from build123d import *

# Parameters (mm, degrees)
SKETCH1_R                                            = 166
SKETCH1_R_2                                          = 131
BOSS_EXTRUDE1_DEPTH                                  = 15
M6_CLEARANCE_HOLE1_D                                 = 6.6
CIRPATTERN1_COUNT                                    = 8
SKETCH4_R                                            = 10
CUT_EXTRUDE1_DEPTH                                   = 4
CSK_FOR_M10_HEX_SOCKET_COUNTERSUNK_CAP_S_D           = 11
CSK_FOR_M10_HEX_SOCKET_COUNTERSUNK_CAP_S_CSINK_D     = 24.4
CSK_FOR_M10_HEX_SOCKET_COUNTERSUNK_CAP_S_CSINK_ANGLE = 90
CIRPATTERN2_COUNT                                    = 4


with BuildPart() as part:
    # Sketch1 → Boss-Extrude1 (new body)
    with BuildSketch(Plane(origin=(0, 0, 0), x_dir=(1, 0, 0), z_dir=(0, 1, 0))):
        Circle(SKETCH1_R)
        Circle(SKETCH1_R_2, mode=Mode.SUBTRACT)
    extrude(amount=BOSS_EXTRUDE1_DEPTH)

    # M6 Clearance Hole1 (through all)
    with Locations(Plane(origin=(0, 0, 0), x_dir=(-1, 0, 0), z_dir=(0, -1, 0))):
        with Locations((0, 153)):
            m6_clearance_hole1 = Hole(M6_CLEARANCE_HOLE1_D / 2)

    # CirPattern1: M6 Clearance Hole1 ×8 about axis
    cirpattern1_axis = Axis((0, 0, 0), (0, 1, 0))
    for i in range(1, CIRPATTERN1_COUNT):
        add(m6_clearance_hole1.rotate(cirpattern1_axis, i * 360 / CIRPATTERN1_COUNT), mode=Mode.SUBTRACT)

    # Sketch4 → Cut-Extrude1 (cut)
    with BuildSketch(Plane.XZ):
        with Locations((-137.196110578, 56.828489706)):
            Circle(SKETCH4_R)
    cut_extrude1 = extrude(amount=-CUT_EXTRUDE1_DEPTH, mode=Mode.SUBTRACT)

    # CSK for M10 Hex Socket Countersunk Cap Screw1 (through all)
    with Locations(Plane(origin=(0, 15, 0), x_dir=(1, 0, 0), z_dir=(0, 1, 0))):
        with Locations((-137.196110578, -56.828489706)):
            csk_for_m10_hex_socket_countersunk_cap_s = CounterSinkHole(CSK_FOR_M10_HEX_SOCKET_COUNTERSUNK_CAP_S_D / 2, CSK_FOR_M10_HEX_SOCKET_COUNTERSUNK_CAP_S_CSINK_D / 2, counter_sink_angle=CSK_FOR_M10_HEX_SOCKET_COUNTERSUNK_CAP_S_CSINK_ANGLE)

    # CirPattern2: Cut-Extrude1, CSK for M10 Hex Socket Countersunk Cap Screw1 ×4 about axis
    cirpattern2_axis = Axis((0, 0, 0), (0, 1, 0))
    for i in range(1, CIRPATTERN2_COUNT):
        add(cut_extrude1.rotate(cirpattern2_axis, i * 360 / CIRPATTERN2_COUNT), mode=Mode.SUBTRACT)
        add(csk_for_m10_hex_socket_countersunk_cap_s.rotate(cirpattern2_axis, i * 360 / CIRPATTERN2_COUNT), mode=Mode.SUBTRACT)


solid = part.part
Geometry check sheet. Reference: the model listing, model coordinates, mm. A direction names the side the tool comes from. Give positions to 0.01 mm unless a question says otherwise; leave off trailing zeros. Order: outer loops, then holes, each group sorted by start corner. A loop starts at its lowest first (then second) coordinate and runs counter-clockwise, first axis right, second up. Notation, with made-up numbers: M -26.5,13 L 29.5,13 A18 cw 29.5,26 Z; hole C 88,78 d9. An arc over 180 degrees is marked long. Use a Markdown table: item, result.
Item 1: Material ranges on line 1 along X through (y, z) = (9.5, 0); line 2 along Z through (x, y) = (107, 13.25); line 3 along Z through (x, y) = (-153, 10), recorded low to high.
Answers follow:
| item | result |
|---|---|
| line 1 | x = -166 to -156.3, -149.7 to -131, 131 to 149.7, 156.3 to 166 |
| line 2 | z = -126.91 to -111.27, -105.11 to -75.58, 75.58 to 105.11, 111.27 to 126.91 |
| line 3 | z = -64.4 to -3.3, 3.3 to 64.4 |
Item 2: Section check B-B (z = 77). Record the cut outline in (x, y).
Answers follow:
| item | result |
|---|---|
| outline | M -147.06,0 L -105.98,0 L -105.98,15 L -147.06,15 Z; M 105.98,0 L 147.06,0 L 147.06,15 L 105.98,15 Z |
Item 3: Depth check by flat-ended pin: P1, Ø14.5, axis at x = 137.2, z = -56.83, coming from the +Y side; P2, Ø10.5, axis at x = 108.19, z = 108.19, coming from the -Y side; P3, Ø5, axis at y = 1.5, z = 40, coming from the -X side; P4, Ø3, axis at x = -126.5, y = 13, coming from the -Z side. Enter the tip coordinate at first touch or a pass-through.
Answers follow:
| item | result |
|---|---|
| P1 | stops at y = 10.05 |
| P2 | stops at y = 0 |
| P3 | stops at x = -161.71 |
| P4 | stops at z = -109.23 |
Item 4: Section check A-A (x = -13). Record the cut outline in (y, z), and give its area (3 significant figures).
Answers follow:
| item | result |
|---|---|
| outline | M 0,-165.49 L 15,-165.49 L 15,-130.35 L 0,-130.35 Z; M 0,130.35 L 15,130.35 L 15,165.49 L 0,165.49 Z |
| area | 1,050 mm2 |
Item 5: Tool access check on faces 4 (the conical face through (135.93, 8.63, -62.52)), 5 (the cylindrical face through (-53, 1.97, -127.96)). Record the directions out of +Z, -Z, +X, -X, +Y, -Y that give a thin tool (end or side, any length) a straight path to the whole face; none if there is none.
Answers follow:
| item | result |
|---|---|
| face 4 | +Y |
| face 5 | -Y |
Item 6: Draft check along Z on faces 1 (the flat face through (-87, 15, -99)), 2 (the cylindrical face through (-136.004, 6.12, 62.198)), 3 (the cylindrical face through (158.334, 7.395, -49.862)). Enter one of: +Z half, -Z half, draft (parallel to the pull), parting line (faces both ways), or undercut.
Answers follow:
| item | result |
|---|---|
| face 1 | draft |
| face 2 | undercut |
| face 3 | parting line |
